```python
from build123d import *

# Parameters (mm, degrees)
SKIZZE1_W                       = 200
SKIZZE1_H                       = 60.5
AUFSATZ_LINEAR_AUSTRAGEN1_DEPTH = 10
SKIZZE2_W                       = 50.5
SKIZZE2_H                       = 40.5
SCHNITT_LINEAR_AUSTRAGEN1_DEPTH = 5
FASE1_SIZE                      = 5
SCHNITT_LINEAR_AUSTRAGEN2_DEPTH = 10


with BuildPart() as part:
    # Skizze1 → Aufsatz-Linear austragen1 (new body)
    with BuildSketch(Plane.XY):
        with Locations((100, 0)):
            Rectangle(SKIZZE1_W, SKIZZE1_H)
    extrude(amount=AUFSATZ_LINEAR_AUSTRAGEN1_DEPTH)

    # Skizze2 → Schnitt-Linear austragen1 (cut)
    with BuildSketch(Plane.XY.offset(10)):
        with Locations((35.25, 0)):
            Rectangle(SKIZZE2_W, SKIZZE2_H)
        with Locations((100, 0)):
            Rectangle(SKIZZE2_W, SKIZZE2_H)
        with Locations((164.75, 0)):
            Rectangle(SKIZZE2_W, SKIZZE2_H)
    extrude(amount=-SCHNITT_LINEAR_AUSTRAGEN1_DEPTH, mode=Mode.SUBTRACT)

    # Fase1
    fase1_edges = [part.edges().sort_by_distance(p)[0] for p in [
        (100, 30.25, 10),
        (0, 0, 10),
        (100, -30.25, 10),
    ]]
    chamfer(fase1_edges, length=FASE1_SIZE)

    # Skizze4 → Schnitt-Linear austragen2 (cut)
    with BuildSketch(Plane.XY.offset(10)):
        Polygon((200, 16.873625745), (194.8, 20.25), (194.8, 5.05), (200, 8.673625745), align=None)
        Polygon((200, -8.426374255), (194.8, -5.05), (194.8, -20.25), (200, -16.626374255), align=None)
    extrude(amount=-SCHNITT_LINEAR_AUSTRAGEN2_DEPTH, mode=Mode.SUBTRACT)


solid = part.part
```
CAD build for the part. Positions are in the model's coordinates, mm. A direction names the side the tool comes from. Coordinates: 2 decimals unless noted, no trailing zeros. Write each loop counter-clockwise with the first axis right and the second up, starting at its lowest first coordinate (ties: lowest second). Pieces come first, ordered by that corner, then holes. Notation, with made-up numbers: (11.5, 22.25) -> (39.5, 22.25) arc R35 ccw to (39.5, 54.25) -> close; hole circle Ø8 at (-20, 56). An arc over 180 degrees is marked (long way). Use CSV: the item, a comma, the result in double quotes. Start each with the question number.
Item 1: Wall check: probe 1 along X at (y, z) = (-14.5, 8.25); probe 2 along X at (y, z) = (-16, 7.5); probe 3 along X at (y, z) = (-14, 3). Give the ranges that are in metal, low to high.
Item 2: Tool access for faces 1 (the flat face through (99, 30.25, 2)), 2 (the flat face through (35, 0, 5)): list every direction of +Z, -Z, +X, -X, +Y, -Y with a clear straight run to the whole face (end or side of a thin tool).
Item 3: Drop flat-ended pins along their axis: P1, Ø1, axis at x = 121, y = 8.5, coming from the -Z side; P2, Ø1, axis at x = 42.5, z = 6.5, coming from the +Y side; P3, Ø2.5, axis at y = 6, z = 8, coming from the -X side; P4, Ø1.5, axis at x = 101, z = 8, coming from the +Y side. Give the stop position or say it passes through.
Item 4: Band-saw the part on B-B, the plane x = 128. Write the cut outline in (y, z).
Item 5: Band-saw the part on C-C, the plane x = 175.5. Write the cut outline in (y, z).
Item 6: Band-saw the part on A-A, the plane z = 8. Write the cut outline in (x, y).
Item 7: Two-plate mould, pull along Y, no slides. Class faces 3 (the flat face through (35, 20.25, 8)), 4 (the flat face through (98.6, 27.715, 7.535)), 5 (the flat face through (99, 0, 0)): +Y half, -Y half, draft (parallel to the pull), parting line (faces both ways), or undercut.
Response values:
1,probe 1,"x = 3.25 to 10, 60.5 to 74.75, 125.25 to 139.5, 190 to 194.8"
1,probe 2,"x = 2.5 to 10, 60.5 to 74.75, 125.25 to 139.5, 190 to 194.8"
1,probe 3,"x = 0 to 194.8"
2,face 1,"+Z, -Z, +X, -X, +Y"
2,face 2,"+Z"
3,P1,"stops at z = 0"
3,P2,"stops at y = 29.25"
3,P3,"stops at x = 1.75"
3,P4,"stops at y = 28"
4,outline,"(-30.25, 0) -> (30.25, 0) -> (30.25, 5) -> (25.25, 10) -> (-25.25, 10) -> (-30.25, 5) -> close"
5,outline,"(-30.25, 0) -> (30.25, 0) -> (30.25, 5) -> (25.25, 10) -> (20.25, 10) -> (20.25, 5) -> (-20.25, 5) -> (-20.25, 10) -> (-25.25, 10) -> (-30.25, 5) -> close"
6,outline,"(3, -27.25) -> (200, -27.25) -> (200, -16.63) -> (194.8, -20.25) -> (194.8, -5.05) -> (200, -8.43) -> (200, 8.67) -> (194.8, 5.05) -> (194.8, 20.25) -> (200, 16.87) -> (200, 27.25) -> (3, 27.25) -> close; hole (10, -20.25) -> (60.5, -20.25) -> (60.5, 20.25) -> (10, 20.25) -> close; hole (74.75, -20.25) -> (125.25, -20.25) -> (125.25, 20.25) -> (74.75, 20.25) -> close; hole (139.5, -20.25) -> (190, -20.25) -> (190, 20.25) -> (139.5, 20.25) -> close"
7,face 3,"undercut"
7,face 4,"+Y half"
7,face 5,"draft"
